Verification items for the finished model (mm, model axes). A direction names the side the tool comes from. Coordinates: 2 decimals unless noted, no trailing zeros. Order: outer loops, then holes, each group sorted by start corner. A loop starts at its lowest first (then second) coordinate and runs counter-clockwise, first axis right, second up.
Q1. Set-up check for faces 5 (the flat face through (-1.27, 76, -17)), 6 (the flat face through (-9, 76, -10.607)), 7 (the flat face through (-12, 0, -19)), 8 (the flat face through (-9, 76, -23.307)), 9 (the flat face through (-9, 75.057, -17)): record each of +Z, -Z, +X, -X, +Y, -Y from which the full face is reachable in a straight line by a thin tool's end or side.
Q2. Draft check along Z on faces 1 (the flat face through (-18, 36, 0)), 2 (the flat face through (-8, 3.175, -19)), 3 (the flat face through (-18, 36, -36.83)), 4 (the cylindrical face through (-12.04, 1.61, -7.42)). Enter one of: pulls with the +Z half, pulls with the -Z half, needs draft (parallel to the pull), parting line crosses it, or undercut.
Q3. Cross-section at B-B, the plane x = -11.43. Record the boundary of the cut face in (y, z) (3 decimals).
Q4. Cross-section at C-C, the plane z = -22. Record the boundary of the cut face in (x, y) (3 decimals), and give its area (3 significant figures).
Q5. Depth check by flat-ended pin: P1, Ø4.5, axis at x = -11.43, z = -10.16, coming from the -Y side; P2, Ø3, axis at x = -10, y = 76.5, coming from the -Z side; P3, Ø4.5, axis at x = -11.43, z = -26.67, coming from the +Y side (3 decimals); P4, Ø3, axis at x = -6, y = 77, coming from the +Z side. Enter the tip coordinate at first touch or a pass-through.
Q6. Thickness scan on line 1 (Z direction, x = -11.43, y = 0.7); line 2 (X direction, y = 1.9, z = -26.67); line 3 (Y direction, x = -10.25, z = -23) (3 decimals). Record the ranges inside material, lowest first.
Q7. Cross-section at A-A, the plane z = -26.67. Record the boundary of the cut face in (x, y) (3 decimals), and give its area (3 significant figures).
Q8. Cross-section at D-D, the plane y = 38. Record the boundary of the cut face in (x, z).
from build123d import *

# Parameters (mm, degrees)
SKETCH1_W                      = 22.86
SKETCH1_H                      = 36.83
BOSS_EXTRUDE1_DEPTH            = 3.175
SKETCH3_W                      = 6.35
SKETCH3_H                      = 36.83
BOSS_EXTRUDE2_DEPTH            = 74.422
SKETCH4_W                      = 12.7
SKETCH4_H                      = 2.54
BOSS_EXTRUDE3_DEPTH            = 15.24
F_2_0_221_DIAMETER_HOLE1_D     = 5.6134
F_2_0_221_DIAMETER_HOLE1_DEPTH = 3.175


with BuildPart() as part:
    # Sketch1 → Boss-Extrude1 (new body)
    with BuildSketch(Plane(origin=(0, 0, 0), x_dir=(1, 0, 0), z_dir=(0, 1, 0))):
        with Locations((-11.43, 18.415)):
            Rectangle(SKETCH1_W, SKETCH1_H)
    extrude(amount=BOSS_EXTRUDE1_DEPTH)

    # Sketch3 → Boss-Extrude2 (add)
    with BuildSketch(Plane(origin=(0, 3.175, 0), x_dir=(1, 0, 0), z_dir=(0, 1, 0))):
        with Locations((-19.685, 18.415)):
            Rectangle(SKETCH3_W, SKETCH3_H)
    extrude(amount=BOSS_EXTRUDE2_DEPTH)

    # Sketch4 → Boss-Extrude3 (add)
    with BuildSketch(Plane(origin=(-16.51, 0, 0), x_dir=(0, 0, -1), z_dir=(1, 0, 0))):
        with Locations((16.956564639, 76.327)):
            Rectangle(SKETCH4_W, SKETCH4_H)
    extrude(amount=BOSS_EXTRUDE3_DEPTH)

    # #2 (0.221) Diameter Hole1
    with Locations(Plane(origin=(0, 0, 0), x_dir=(-1, 0, 0), z_dir=(0, -1, 0))):
        with Locations((11.43, 10.16), (11.43, 26.67)):
            Hole(F_2_0_221_DIAMETER_HOLE1_D / 2, depth=F_2_0_221_DIAMETER_HOLE1_DEPTH)


solid = part.part
Check values:
1. face 5: +Z, -Z, +X, +Y
1. face 6: +Z, +X, +Y
1. face 7: +Z, -Z, +X, -X, -Y
1. face 8: -Z, +X, +Y
1. face 9: +Z, -Z, +X
2. face 1: pulls with the +Z half
2. face 2: needs draft
2. face 3: pulls with the -Z half
2. face 4: undercut
3. outline: (0, -36.83) - (3.175, -36.83) - (3.175, -29.477) - (0, -29.477) - close; (0, -23.863) - (3.175, -23.863) - (3.175, -12.967) - (0, -12.967) - close; (0, -7.353) - (3.175, -7.353) - (3.175, 0) - (0, 0) - close; (75.057, -23.307) - (77.597, -23.307) - (77.597, -10.607) - (75.057, -10.607) - close
4. outline: (-22.86, 0) - (0, 0) - (0, 3.175) - (-16.51, 3.175) - (-16.51, 75.057) - (-1.27, 75.057) - (-1.27, 77.597) - (-22.86, 77.597) - close
4. area: 584 mm2
5. P1: stops at y = 75.06
5. P2: stops at z = -23.31
5. P3: passes through
5. P4: stops at z = -10.61
6. line 1: z = -36.83 to -29.48, -23.86 to -12.97, -7.35 to 0
6. line 2: x = -22.86 to -14.24, -8.62 to 0
6. line 3: y = 0 to 3.175, 75.057 to 77.597
7. outline: (-22.86, 0) - (-14.237, 0) - (-14.237, 3.175) - (-16.51, 3.175) - (-16.51, 77.597) - (-22.86, 77.597) - close; (-8.623, 0) - (0, 0) - (0, 3.175) - (-8.623, 3.175) - close
7. area: 527 mm2
8. outline: (-22.86, -36.83) - (-16.51, -36.83) - (-16.51, 0) - (-22.86, 0) - close
